The model under review builds one solid part; all positions refer to its coordinate system, in mm. Round coordinates to 2 decimals unless told otherwise and drop trailing zeros. Order: outer loops, then holes, each group sorted by start corner. A loop starts at its lowest first (then second) coordinate and runs counter-clockwise, first axis right, second up. Notation, with made-up numbers: (34, 53.5) -> (68, 53.5) arc R17 cw to (68, 80.5) -> close; hole circle Ø2 at (80, 28). An arc over 180 degrees is marked (long way). Use a Markdown table: item, result. Add a question column.
```python
from build123d import *

# Parameters (mm, degrees)
SKETCH1_W            = 635.3556
SKETCH1_H            = 165.1
BOSS_EXTRUDE1_DEPTH  = 1.5875
SKETCH2_W            = 254
SKETCH2_H            = 3.175
BOSS_EXTRUDE2_DEPTH  = 3.175
BOSS_EXTRUDE3_DEPTH  = 3.175
SKETCH5_W            = 3.175
SKETCH5_H            = 76.2
SKETCH5_W_2          = 2.286
SKETCH5_H_2          = 107.442
CUT_EXTRUDE2_DEPTH   = 4.175
M6_CLEARANCE_HOLE1_D = 6.6
LPATTERN2_COUNT      = 4
LPATTERN2_PITCH      = 177.8


with BuildPart() as part:
    # Sketch1 → Boss-Extrude1 (new body, symmetric)
    with BuildSketch(Plane(origin=(0, 0, 0), x_dir=(1, 0, 0), z_dir=(0, 1, 0))):
        Rectangle(SKETCH1_W, SKETCH1_H)
    extrude(amount=BOSS_EXTRUDE1_DEPTH, both=True)

    # Sketch2 → Boss-Extrude2 (add)
    with BuildSketch(Plane(origin=(0, 0, -82.55), x_dir=(-1, 0, 0), z_dir=(0, 0, -1))):
        with Locations((-157.8229, 0)):
            Rectangle(SKETCH2_W, SKETCH2_H)
        with Locations((157.8229, 0)):
            Rectangle(SKETCH2_W, SKETCH2_H)
    extrude(amount=BOSS_EXTRUDE2_DEPTH)

    # Sketch3 → Boss-Extrude3 (add)
    with BuildSketch(Plane.XZ.offset(1.5875)):
        Polygon((317.6778, -82.55), (352.6028, -82.55), (352.6028, -79.375), (317.6778, -34.925), align=None)
    boss_extrude3 = extrude(amount=-BOSS_EXTRUDE3_DEPTH)

    # Mirror1: Boss-Extrude3 across plane
    add(boss_extrude3.mirror(Plane(origin=(0, 0, 0), x_dir=(0, 0, 1), z_dir=(1, 0, 0))))

    # Sketch5 → Cut-Extrude2 (cut, through all)
    with BuildSketch(Plane.XZ.offset(1.5875)):
        with Locations((316.0903, 44.45)):
            Rectangle(SKETCH5_W, SKETCH5_H)
        with Locations((-316.0903, 44.45)):
            Rectangle(SKETCH5_W, SKETCH5_H)
        with Locations((0, -28.829)):
            Rectangle(SKETCH5_W_2, SKETCH5_H_2)
    extrude(amount=-CUT_EXTRUDE2_DEPTH, mode=Mode.SUBTRACT)

    # M6 Clearance Hole1 (through all)
    with Locations(Plane(origin=(0, 1.5875, 0), x_dir=(1, 0, 0), z_dir=(0, 1, 0))):
        with Locations((266.7, -73.8124)):
            m6_clearance_hole1 = Hole(M6_CLEARANCE_HOLE1_D / 2)

    # LPattern2: M6 Clearance Hole1 ×4
    with Locations(*[(-i * LPATTERN2_PITCH, 0, 0) for i in range(1, LPATTERN2_COUNT)]):
        add(m6_clearance_hole1, mode=Mode.SUBTRACT)


solid = part.part
```
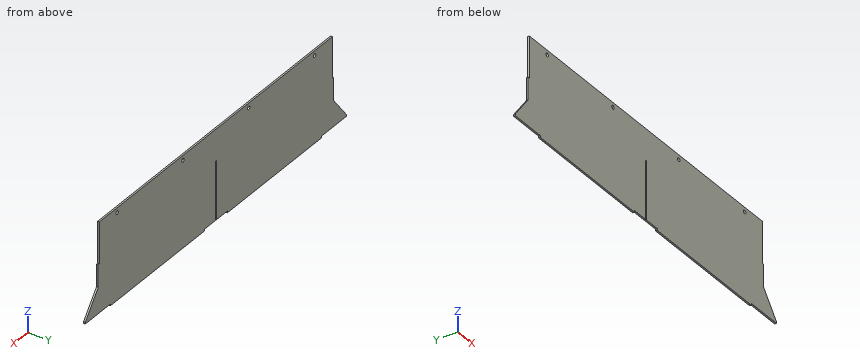
Q1. Add section D-D, the plane z = 64.5. Give the boundary of the cut face in (x, y), then the cut area to 3 significant figures.
Q2. To check wall thickness, follow line 1 along X through (y, z) = (0, 74); line 2 along X through (y, z) = (-0.95, 7); line 3 along Z through (x, y) = (-266.7, 0.8) (3 decimals). State the ranges of each line that lie inside material, in increasing order.
Q3. Add section B-B, the plane z = -41.5. Give the boundary of the cut face in (x, y).
Q4. For pin 1 (1 mm diameter, centred on x = 330.5, y = 0.5, fed in from -Z); pin 2 (6 mm diameter, centred on x = 266.7, z = 73.81, fed in from +Y); pin 3 (0.7 mm diameter, centred on x = 0, y = 0.5, fed in from -Z); pin 4 (1 mm diameter, centred on x = 316.5, y = -0.5, fed in from +Z), all flat-tipped, find the tip position at first contact; note any pin that passes through.
Q5. Add section A-A, the plane y = -1.1. Give the boundary of the cut face in (x, z) (3 decimals).
Q6. Add section C-C, the plane x = -13.5. Give the boundary of the cut face in (y, z).
Return value:
| question | item | result |
|---|---|---|
| 1 | outline | (-314.5, -1.59) -> (314.5, -1.59) -> (314.5, 1.59) -> (-314.5, 1.59) -> close |
| 1 | area | 2,000 mm² |
| 2 | line 1 | -314.5 to -269.99, -263.41 to -92.19, -85.61 to 85.61, 92.19 to 263.41, 269.99 to 314.5 |
| 2 | line 2 | -314.5 to -1.14, 1.14 to 314.5 |
| 2 | line 3 | -85.725 to 70.512, 77.112 to 82.55 |
| 3 | outline | (-322.84, -1.59) -> (-1.14, -1.59) -> (-1.14, 1.59) -> (-322.84, 1.59) -> close; (1.14, -1.59) -> (322.84, -1.59) -> (322.84, 1.59) -> (1.14, 1.59) -> close |
| 4 | pin 1 | z = -82.55 |
| 4 | pin 2 | through |
| 4 | pin 3 | z = 24.89 |
| 4 | pin 4 | z = 6.35 |
| 5 | outline | (-352.603, -82.55) -> (-284.823, -82.55) -> (-284.823, -85.725) -> (-30.823, -85.725) -> (-30.823, -82.55) -> (-1.143, -82.55) -> (-1.143, 24.892) -> (1.143, 24.892) -> (1.143, -82.55) -> (30.823, -82.55) -> (30.823, -85.725) -> (284.823, -85.725) -> (284.823, -82.55) -> (352.603, -82.55) -> (352.603, -79.375) -> (317.678, -34.925) -> (317.678, 6.35) -> (314.503, 6.35) -> (314.503, 82.55) -> (-314.503, 82.55) -> (-314.503, 6.35) -> (-317.678, 6.35) -> (-317.678, -34.925) -> (-352.603, -79.375) -> close; hole circle Ø6.6 at (-266.7, 73.812); hole circle Ø6.6 at (-88.9, 73.812); hole circle Ø6.6 at (88.9, 73.812); hole circle Ø6.6 at (266.7, 73.812) |
| 6 | outline | (-1.59, -82.55) -> (1.59, -82.55) -> (1.59, 82.55) -> (-1.59, 82.55) -> close |
